from build123d import *

# Parameters (mm, degrees)
F0_R     = 1.5
F0_R_2   = 4.5
F0_W     = 9
F0_H     = 5
F0_W_2   = 38
F0_H_2   = 42
F0_W_3   = 22
F0_H_3   = 18
F1_DEPTH = 1.5
F2_R     = 5
F3_R     = 8.99999


# Not quite as in the source:
# - a fillet or chamfer is up to 0.001 mm smaller than in the source, because OpenCascade refuses the exact size


with BuildPart() as f1:
    # F0 (on Top) → F1 (new body)
    with BuildSketch(Plane.XY):
        Polygon((-77.5, -42.5), (77.5, -42.5), (77.5, 42.5), (-77.5, 42.5), (-77.5, 9), (-77.5, -9), align=None)
        with Locations((-72, -38)):
            Circle(F0_R, mode=Mode.SUBTRACT)
        Polygon((-49.4840586844, -25.6258432192), (-64.3245950341, -36.0181480646), (-64.3245950341, -25.6258432192), align=None, mode=Mode.SUBTRACT)
        with Locations((-72, -23)):
            Circle(F0_R, mode=Mode.SUBTRACT)
        with Locations((-20, -38)):
            Circle(F0_R, mode=Mode.SUBTRACT)
        with Locations((-40, -28)):
            Circle(F0_R_2, mode=Mode.SUBTRACT)
        with Locations((-20, -28)):
            Circle(F0_R_2, mode=Mode.SUBTRACT)
        with Locations((-72, -10)):
            Circle(F0_R, mode=Mode.SUBTRACT)
        Polygon((-49.4840586844, -13.3469680754), (-64.3245950341, -5.3528225981), (-49.4840586844, -5.3528225981), align=None, mode=Mode.SUBTRACT)
        Polygon((-43.9106635749, -19.5035282522), (-43.9106635749, -5.3528225981), (-27.3078400642, -5.3528225981), align=None, mode=Mode.SUBTRACT)
        with Locations((20, -38)):
            Circle(F0_R, mode=Mode.SUBTRACT)
        with Locations((0, -28)):
            Circle(F0_R_2, mode=Mode.SUBTRACT)
        with Locations((20, -28)):
            Circle(F0_R_2, mode=Mode.SUBTRACT)
        with Locations((72, -38)):
            Circle(F0_R, mode=Mode.SUBTRACT)
        with Locations((40, -28)):
            Circle(F0_R_2, mode=Mode.SUBTRACT)
        Polygon((64.3245950341, -36.0181480646), (49.4840586844, -25.6258432192), (64.3245950341, -25.6258432192), align=None, mode=Mode.SUBTRACT)
        with Locations((72, -23)):
            Circle(F0_R, mode=Mode.SUBTRACT)
        Polygon((43.9106635749, -19.5035282522), (27.3078400642, -5.3528225981), (43.9106635749, -5.3528225981), align=None, mode=Mode.SUBTRACT)
        Polygon((64.3245950341, -5.3528225981), (49.4840586844, -13.3469680754), (49.4840586844, -5.3528225981), align=None, mode=Mode.SUBTRACT)
        with Locations((72, -10)):
            Circle(F0_R, mode=Mode.SUBTRACT)
        with Locations((-74.5, 0)):
            Circle(F0_R, mode=Mode.SUBTRACT)
        with Locations((-66.3017949164, 0)):
            Rectangle(F0_W, F0_H, mode=Mode.SUBTRACT)
        with Locations((-59.5, 0)):
            Circle(F0_R, mode=Mode.SUBTRACT)
        with Locations((-72, 10)):
            Circle(F0_R, mode=Mode.SUBTRACT)
        Polygon((-49.4840586844, 5.3528225981), (-64.3245950341, 5.3528225981), (-49.4840586844, 13.3469680754), align=None, mode=Mode.SUBTRACT)
        Polygon((-43.9106635749, 5.3528225981), (-43.9106635749, 19.5035282522), (-27.3078400642, 5.3528225981), align=None, mode=Mode.SUBTRACT)
        with Locations((-72, 23)):
            Circle(F0_R, mode=Mode.SUBTRACT)
        Polygon((-64.3245950341, 36.0181480646), (-49.4840586844, 25.6258432192), (-64.3245950341, 25.6258432192), align=None, mode=Mode.SUBTRACT)
        with Locations((-72, 38)):
            Circle(F0_R, mode=Mode.SUBTRACT)
        with Locations((-40, 28)):
            Circle(F0_R_2, mode=Mode.SUBTRACT)
        with Locations((-20, 28)):
            Circle(F0_R_2, mode=Mode.SUBTRACT)
        with Locations((-20, 38)):
            Circle(F0_R, mode=Mode.SUBTRACT)
        Rectangle(F0_W_2, F0_H_2, mode=Mode.SUBTRACT)
        Polygon((49.4840586844, 5.3528225981), (49.4840586844, 13.3469680754), (64.3245950341, 5.3528225981), align=None, mode=Mode.SUBTRACT)
        with Locations((72, 10)):
            Circle(F0_R, mode=Mode.SUBTRACT)
        Polygon((43.9106635749, 19.5035282522), (43.9106635749, 5.3528225981), (27.3078400642, 5.3528225981), align=None, mode=Mode.SUBTRACT)
        with Locations((0, 28)):
            Circle(F0_R_2, mode=Mode.SUBTRACT)
        with Locations((20, 28)):
            Circle(F0_R_2, mode=Mode.SUBTRACT)
        with Locations((20, 38)):
            Circle(F0_R, mode=Mode.SUBTRACT)
        with Locations((40, 28)):
            Circle(F0_R_2, mode=Mode.SUBTRACT)
        with Locations((72, 23)):
            Circle(F0_R, mode=Mode.SUBTRACT)
        Polygon((64.3245950341, 25.6258432192), (49.4840586844, 25.6258432192), (64.3245950341, 36.0181480646), align=None, mode=Mode.SUBTRACT)
        with Locations((72, 38)):
            Circle(F0_R, mode=Mode.SUBTRACT)
        with Locations((-88.5, 0)):
            Rectangle(F0_W_3, F0_H_3)
        with Locations((-95.5, 0)):
            Circle(F0_R, mode=Mode.SUBTRACT)
        with Locations((-88.6982050836, 0)):
            Rectangle(F0_W, F0_H, mode=Mode.SUBTRACT)
        with Locations((-80.5, 0)):
            Circle(F0_R, mode=Mode.SUBTRACT)
    extrude(amount=F1_DEPTH)

    # F2
    f2_edges = [f1.edges().sort_by_distance(p)[0] for p in [
        (-77.5, 42.5, 0.75),
        (77.5, 42.5, 0.75),
        (77.5, -42.5, 0.75),
        (-77.5, -42.5, 0.75),
    ]]
    fillet(f2_edges, radius=F2_R)

    # F3 (radius 9 in the source; OpenCascade refuses exactly that, so slightly less here)
    f3_edges = [f1.edges().sort_by_distance(p)[0] for p in [
        (-77.5, -9, 0.75),
        (-77.5, 9, 0.75),
        (-99.5, -9, 0.75),
        (-99.5, 9, 0.75),
    ]]
    fillet(f3_edges, radius=F3_R)


solid = f1.part
Source: CAD feature listing. Evaluate the final solid. Frame: model axes, mm. Round coordinates to 2 decimals unless told otherwise and drop trailing zeros. Loops run counter-clockwise (first coordinate to the right, second up) from the corner with the lowest first, then second, coordinate; pieces in that order, holes last.
Q1. Section D-D, the plane x = 57.5. Return loops of the section in (y, z).
Q2. Section C-C, the plane z = 0.7. State how many separate pieces and enclosed holes the cut face has, plus the area to 3 significant figures.
Q3. Ray query, line 1 (Y direction, x = -20, z = 0.7); line 2 (Y direction, x = 0, z = 1.25); line 3 (Y direction, x = 40.5, z = 1.4). Return the intervals inside material, ascending.
Q4. Section A-A, the plane x = 12.5. Return loops of the section in (y, z), plus the area to 3 significant figures.
Q5. Section B-B, the plane x = -52. Return loops of the section in (y, z), plus the area to 3 significant figures.
Q6. Mould query, pull axis X, two halves, no side actions, for faces 1 (the face through (27, 1, 0)), 2 (the face through (76, -41.07, 0.76)), 3 (the face through (35.493, 12.329, 0.74)). Classes: pulls with the +X half, pulls with the -X half, needs draft (parallel to the pull), parting line crosses it, or undercut.
Solutions:
1. outline: (-42.5, 0) - (-31.24, 0) - (-31.24, 1.5) - (-42.5, 1.5) - close; (-25.63, 0) - (-9.03, 0) - (-9.03, 1.5) - (-25.63, 1.5) - close; (-5.35, 0) - (5.35, 0) - (5.35, 1.5) - (-5.35, 1.5) - close; (9.03, 0) - (25.63, 0) - (25.63, 1.5) - (9.03, 1.5) - close; (31.24, 0) - (42.5, 0) - (42.5, 1.5) - (31.24, 1.5) - close
2. separate pieces: 1
2. enclosed holes: 45
2. area: 10,100 mm2
3. line 1: y = -42.5 to -39.5, -36.5 to -32.5, -23.5 to 23.5, 32.5 to 36.5, 39.5 to 42.5
3. line 2: y = -42.5 to -32.5, -23.5 to -21, 21 to 23.5, 32.5 to 42.5
3. line 3: y = -42.5 to -32.47, -23.53 to -16.6, -5.35 to 5.35, 16.6 to 23.53, 32.47 to 42.5
4. outline: (-42.5, 0) - (-21, 0) - (-21, 1.5) - (-42.5, 1.5) - close; (21, 0) - (42.5, 0) - (42.5, 1.5) - (21, 1.5) - close
4. area: 64.5 mm2
5. outline: (-42.5, 0) - (-27.39, 0) - (-27.39, 1.5) - (-42.5, 1.5) - close; (-25.63, 0) - (-11.99, 0) - (-11.99, 1.5) - (-25.63, 1.5) - close; (-5.35, 0) - (5.35, 0) - (5.35, 1.5) - (-5.35, 1.5) - close; (11.99, 0) - (25.63, 0) - (25.63, 1.5) - (11.99, 1.5) - close; (27.39, 0) - (42.5, 0) - (42.5, 1.5) - (27.39, 1.5) - close
5. area: 102 mm2
6. face 1: needs draft
6. face 2: pulls with the +X half
6. face 3: undercut
